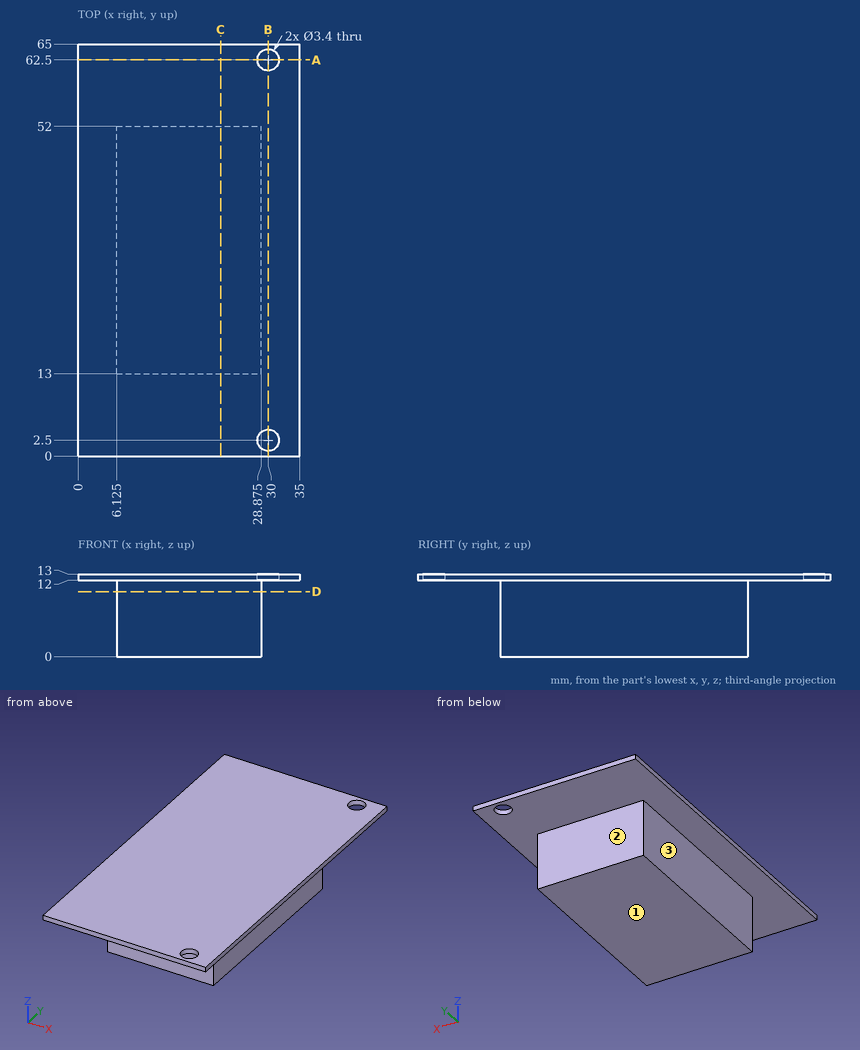
Design review of the part shown in the three views and the two pictorial views. Dimensions are in mm from the part's minimum x, y and z. A direction names the side the tool comes from. Coordinates: 2 decimals unless noted, no trailing zeros. Loops run counter-clockwise (first coordinate to the right, second up) from the corner with the lowest first, then second, coordinate; pieces in that order, holes last. Notation, with made-up numbers: (9.25, 58.5) - (53.25, 58.5) arc R16 ccw to (53.25, 77.5) - close; hole circle Ø3 at (40.5, 38). An arc over 180 degrees is marked (long way). Use a Markdown table: item, result. Add a question column.
Item 1: Insertion check: pin 1 Ø5 at (y, z) = (8.5, 7) entering from +X; pin 2 Ø1.5 at (x, z) = (12.5, 4) entering from -Y; pin 3 Ø6 at (y, z) = (40.5, 5) entering from -X (3 decimals); pin 4 Ø3.5 at (x, z) = (14.5, 8.5) entering from +Y. Each pin has a flat end and moves straight along its axis. Give the tip position at first contact, or say it passes through.
Item 2: Tool access review of the marked faces 1, 2 and 3: name each direction out of +Z, -Z, +X, -X, +Y, -Y from which nothing blocks a thin tool from reaching the whole face with its end or side.
Item 3: We need section A-A (y = 62.5). Give the boundary of the cut face in (x, z).
Item 4: We need section D-D (z = 10.25). Give the boundary of the cut face in (x, y) (3 decimals).
Item 5: We need section B-B (x = 30). Give the boundary of the cut face in (y, z), and give its area (3 significant figures).
Item 6: We need section C-C (x = 22.5). Give the boundary of the cut face in (y, z), and give its area (3 significant figures).
Item 7: For line 1 (Y direction, x = 30, z = 12.7); line 2 (Y direction, x = 6.5, z = 9); line 3 (X direction, y = 19, z = 10) (3 decimals), list the stretches that pass through material, from the lowest coordinate up.
Results list:
| question | item | result |
|---|---|---|
| 1 | pin 1 | passes through |
| 1 | pin 2 | stops at y = 13 |
| 1 | pin 3 | stops at x = 6.125 |
| 1 | pin 4 | stops at y = 52 |
| 2 | face 1 | -Z, +X, -X, +Y, -Y |
| 2 | face 2 | -Z, +X, -X, +Y |
| 2 | face 3 | -Z, -X, +Y, -Y |
| 3 | outline | (0, 12) - (28.3, 12) - (28.3, 13) - (0, 13) - close; (31.7, 12) - (35, 12) - (35, 13) - (31.7, 13) - close |
| 4 | outline | (6.125, 13) - (28.875, 13) - (28.875, 52) - (6.125, 52) - close |
| 5 | outline | (0, 12) - (0.8, 12) - (0.8, 13) - (0, 13) - close; (4.2, 12) - (60.8, 12) - (60.8, 13) - (4.2, 13) - close; (64.2, 12) - (65, 12) - (65, 13) - (64.2, 13) - close |
| 5 | area | 58.2 mm^2 |
| 6 | outline | (0, 12) - (13, 12) - (13, 0) - (52, 0) - (52, 12) - (65, 12) - (65, 13) - (0, 13) - close |
| 6 | area | 533 mm^2 |
| 7 | line 1 | y = 0 to 0.8, 4.2 to 60.8, 64.2 to 65 |
| 7 | line 2 | y = 13 to 52 |
| 7 | line 3 | x = 6.125 to 28.875 |
